```python
from build123d import *

# Parameters (mm, degrees)
F1_DEPTH = 16.6271422058
F2_R     = 2.54
F3_DEPTH = 20.8997240989
F4_SIZE2 = 0.508
F4_SIZE  = 0.508


with BuildPart() as f1:
    # F0 (on Top) → F1 (new body)
    with BuildSketch(Plane.XY):
        with BuildLine():
            Line((-36.148622632, 0), (0, -46.8087121844))
            Line((0, -46.8087121844), (36.148622632, 0))
            ThreePointArc((36.148622632, 0), (31.497984523, 31.6851542178), (0, 25.9011760354))
            ThreePointArc((0, 25.9011760354), (-31.497984523, 31.6851542178), (-36.148622632, 0))
        make_face()
    extrude(amount=F1_DEPTH)

    # F2
    f2_edges = [f1.edges().sort_by_distance(p)[0] for p in [
        (-31.497985, 31.685154, 16.627142),
        (-18.074311, -23.404356, 16.627142),
        (18.074311, -23.404356, 16.627142),
        (31.497985, 31.685154, 16.627142),
    ]]
    fillet(f2_edges, radius=F2_R)

    # F3 (add): a face of the model
    f3_faces = [f1.faces().sort_by_distance(p)[0] for p in [
        (0, 3.7630845429, 16.6271422058),
    ]]
    extrude(f3_faces, amount=-F3_DEPTH)

    # F4
    f4_edges = [f1.edges().sort_by_distance(p)[0] for p in [
        (-28.022292, 30.877177, -4.272582),
        (28.022292, 30.877177, -4.272582),
        (-17.069153, -20.550289, -4.272582),
        (17.069153, -20.550289, -4.272582),
    ]]
    chamfer(f4_edges, length=F4_SIZE, length2=F4_SIZE2)


solid = f1.part
```
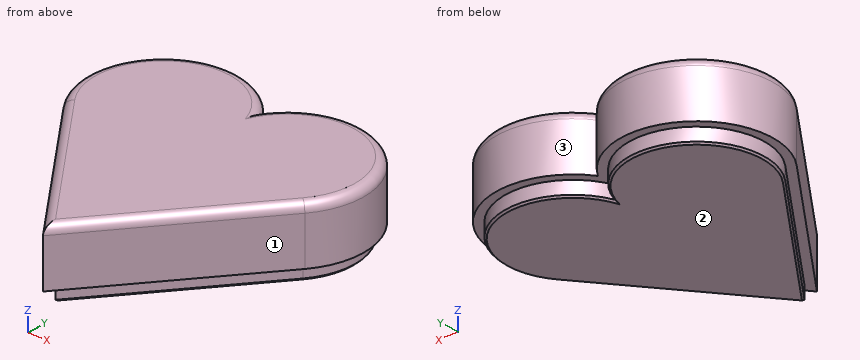
Design review of the part built by this model. Coordinates are the model's own, in mm. Face numbers are marked on the shaded views. Give positions to 0.01 mm unless a question says otherwise; leave off trailing zeros. Write each loop counter-clockwise with the first axis right and the second up, starting at its lowest first coordinate (ties: lowest second). Pieces come first, ordered by that corner, then holes.
(1) Clearance check with flat-ended pins moving along their axes: pin 1 Ø3 at (y, z) = (-31.5, 2.5) entering from -X; pin 2 Ø1 at (x, z) = (-8, 9) entering from -Y; pin 3 Ø6 at (x, z) = (25.5, 12.5) entering from -Y. State where each tip first meets the part, or that it passes through.
Checked values:
pin 1: stops at x = -12.98
pin 2: stops at y = -37.1
pin 3: stops at y = -17.67
(2) Add section A-A (z = 10.5). Give the boundary of the cut face in (x, y), and give its area (3 significant figures).
Checked values:
outline: (-36.15, 0) - (0, -46.81) - (36.15, 0) arc R22.25 ccw (long way) to (0, 25.9) arc R22.25 ccw (long way) to start
area: 4,250 mm2
(3) Mouldability with a two-part tool opening along X and no side actions: class the marked faces 1, 2 and 3 as +X half, -X half, draft (parallel to the pull), parting line (faces both ways), or undercut.
Checked values:
face 1: +X half
face 2: draft
face 3: undercut
(4) Wall thickness on line 1 along X through (y, z) = (29, 5.5); line 2 along Y through (x, z) = (-19, 12); line 3 along Y through (x, z) = (-15, -2.75): over which ranges is each line inside the solid? List them lowest first.
Checked values:
line 1: x = -34.6 to -2.48, 2.48 to 34.6
line 2: y = -22.21 to 35.84
line 3: y = -23.23 to 32.99
